Build history of the part. All positions in model axes, mm. A direction names the side the tool comes from. Coordinates: 2 decimals unless noted, no trailing zeros. Write each loop counter-clockwise with the first axis right and the second up, starting at its lowest first coordinate (ties: lowest second). Pieces come first, ordered by that corner, then holes. Notation, with made-up numbers: M -6.75,-37 L 18.25,-37 A35 cw 18.25,-3 Z; hole C -16.75,34.25 d2. An arc over 180 degrees is marked long. Use CSV: the item, a comma, the result in double quotes. Start each with the question number.
Autodesk Fusion 360 part; units mm, degrees
sketch "Sketch1" plane through (0, 0, 0) normal (0, 0, 1) x (1, 0, 0)
  line L0 (31.5, -7) -> (-31.5, -7)
  line L1 (-31.5, -7) -> (-31.5, 7)
  line L2 (-31.5, 7) -> (31.5, 7)
  line L3 (31.5, 7) -> (31.5, -7)
  line L4 (31.5, -7) -> (-31.5, 7) construction
  line L5 (-31.5, -7) -> (31.5, 7) construction
  dimension "d1" = 63
  dimension "d2" = 14
extrude "Extrude1" add sketch "Sketch1" along normal blind 2 makes body 1
sketch "Sketch3" plane through (0, 0, 2) normal (0, 0, 1) x (-1, 0, 0)
  line L0 (-31.5, -7) -> (31.5, -7)
  line L1 (31.5, -7) -> (31.5, 7)
  line L2 (31.5, 7) -> (-31.5, 7)
  line L3 (-31.5, 7) -> (-31.5, -7)
  line L4 (25.5, 0.7) -> (-25.5, 0.7)
  line L5 (-25.5, 0.7) -> (-25.5, -0.7)
  line L6 (-25.5, -0.7) -> (25.5, -0.7)
  line L7 (25.5, -0.7) -> (25.5, 0.7)
  line L8 (25.5, 0.7) -> (-25.5, -0.7) construction
  line L9 (-25.5, 0.7) -> (25.5, -0.7) construction
  line L10 (-27.5, 2.7) -> (27.5, 2.7)
  line L11 (27.5, 2.7) -> (27.5, -2.7)
  line L12 (27.5, -2.7) -> (-27.5, -2.7)
  line L13 (-27.5, -2.7) -> (-27.5, 2.7)
  line L14 (-27.5, 2.7) -> (27.5, -2.7) construction
  line L15 (27.5, 2.7) -> (-27.5, -2.7) construction
  dimension "d7" = 51
  dimension "d8" = 1.4
  dimension "d9" = 55
  dimension "d10" = 5.4
extrude "Extrude2" add sketch "Sketch3" along normal blind 13 contours L10 L11 L12 L13 bodies 1
fillet "Fillet1" radius 1 4 edges at (-27.5, -2.7, 8.5) (27.5, -2.7, 8.5) (-27.5, 2.7, 8.5) (27.5, 2.7, 8.5) on bodies 1
fillet "Fillet2" radius 2 4 edges at (-31.5, 7, 1) (31.5, 7, 1) (31.5, -7, 1) (-31.5, -7, 1) on bodies 1
copy_body "Body->Comp1" bodies 1 removing the originals makes body 2 in component "Grating_Holder"
component "Grating_Holder" placed x (1, 0, 0) y (0, 1, 0) z (0, 0, 1) at (0, 0, 0)
1. Flat gauge pins, fed straight in: pin 1 (2 mm diameter, centred on x = -7.5, z = 11.5, fed in from -Y); pin 2 (0.7 mm diameter, centred on y = 0, z = 8.5, fed in from -X); pin 3 (5 mm diameter, centred on x = 8.5, z = 6.5, fed in from +Y). Where does each tip first touch, or does it go through?
2. 3-axis set-ups, long thin cutter, end or side, ignore diameter. For faces 1 (the flat face through (-25.5, 0, 8)), 2 (the cylindrical face through (27.215, 2.399, 8.591)), 3 (the cylindrical face through (-27.199, 2.415, 8.591)), 4 (the flat face through (-27.5, 0, 8)): which of +Z, -Z, +X, -X, +Y, -Y reach the whole face in a straight line?
3. Slice it at D-D (y = 6). List the corners of the cut face in (x, z).
4. Slice it at A-A (x = -9). List the corners of the cut face in (y, z).
5. Drill centre lines: line 1 along Y through (x, z) = (16.5, 3.25); line 2 along Z through (x, y) = (22, 4); line 3 along X through (y, z) = (0.75, 3). Where is each one in solid material? Low to high. Write a range as from..to.
6. Slice it at B-B (z = 3.25). List the corners of the cut face in (x, y).
7. Slice it at C-C (y = -4). List the corners of the cut face in (x, z).
8. Pull direction X, two halves, no side cores. Call faces 5 (the cylindrical face through (30.93, 6.4, 1.01)), 6 (the flat face through (0, 0, 2)), 7 (the flat face through (0, -2.7, 8)): pulls with the +X half, pulls with the -X half, needs draft (parallel to the pull), parting line crosses it, or undercut.
Established:
1,pin 1,"stops at y = -2.7"
1,pin 2,"stops at x = -27.5"
1,pin 3,"stops at y = 2.7"
2,face 1,"+Z"
2,face 2,"+Z, +X, +Y"
2,face 3,"+Z, -X, +Y"
2,face 4,"+Z, -X, +Y, -Y"
3,outline,"M -31.23,0 L 31.23,0 L 31.23,2 L -31.23,2 Z"
4,outline,"M -7,0 L 7,0 L 7,2 L 2.7,2 L 2.7,15 L 0.7,15 L 0.7,2 L -0.7,2 L -0.7,15 L -2.7,15 L -2.7,2 L -7,2 Z"
5,line 1,"y = -2.7..-0.7, 0.7..2.7"
5,line 2,"z = 0..2"
5,line 3,"x = -27.5..27.5"
6,outline,"M -27.5,-1.7 A1 ccw -26.5,-2.7 L 26.5,-2.7 A1 ccw 27.5,-1.7 L 27.5,1.7 A1 ccw 26.5,2.7 L -26.5,2.7 A1 ccw -27.5,1.7 Z; hole M -25.5,-0.7 L 25.5,-0.7 L 25.5,0.7 L -25.5,0.7 Z"
7,outline,"M -31.5,0 L 31.5,0 L 31.5,2 L -31.5,2 Z"
8,face 5,"pulls with the +X half"
8,face 6,"undercut"
8,face 7,"needs draft"
